Could you check a few things on this model? Use its own coordinates, in mm. Give positions to 0.01 mm unless a question says otherwise; leave off trailing zeros. Loops run counter-clockwise (first coordinate to the right, second up) from the corner with the lowest first, then second, coordinate; pieces in that order, holes last. Notation, with made-up numbers: (26, -37) - (35, -37) arc R21 ccw to (35, -9) - close; hole circle Ø4 at (-18, 71). An arc over 180 degrees is marked (long way). Write each question's results on one line, items separated by ' | '. Start each with the question number.
(1) Suppose I cut it at A-A (y = 0). Count the separate pieces of the cut face and the enclosed holes in it, and give its area (3 significant figures).
(2) Suppose I cut it at B-B (x = 25.4). Please give me the cut outline in (y, z), and give its area (3 significant figures).
(3) For pin 1 (1.2 mm diameter, centred on x = 20, z = -0.5, fed in from +Y); pin 2 (1.2 mm diameter, centred on y = 25, z = -0.5, fed in from +X); pin 3 (1.2 mm diameter, centred on y = 27.5, z = 0.5, fed in from -X), each with a flat end and sliding along its axis, tell me the tip position at first contact or that it passes through.
(4) I need wall thicknesses on line 1 (Y direction, x = 0, z = 0); line 2 (Y direction, x = 1.5, z = -0.5); line 3 (Y direction, x = 21, z = 0.95). Which ranges of each line are inside material? Lowest first, please.
from build123d import *

# Parameters (mm, degrees)
SKETCH1_R           = 2.5
BOSS_EXTRUDE1_DEPTH = 2.5


with BuildPart() as part:
    # Sketch1 → Boss-Extrude1 (new body)
    with BuildSketch(Plane(origin=(0, 0, -1.25), x_dir=(-1, 0, 0), z_dir=(0, 0, -1))):
        Polygon((12.7, 12.7), (12.7, 50.546), (6.35, 56.896), (-6.35, 56.896), (-12.7, 50.546), (-12.7, 12.7), (-37.846, 12.7), (-44.196, 6.35), (-44.196, -6.35), (-37.846, -12.7), (37.846, -12.7), (44.196, -6.35), (44.196, 6.35), (37.846, 12.7), align=None)
        with Locations((0, 50.8)):
            Circle(SKETCH1_R, mode=Mode.SUBTRACT)
        with Locations((0, 38.1)):
            Circle(SKETCH1_R, mode=Mode.SUBTRACT)
        with Locations((-38.1, 0)):
            Circle(SKETCH1_R, mode=Mode.SUBTRACT)
        with Locations((-25.4, 0)):
            Circle(SKETCH1_R, mode=Mode.SUBTRACT)
        with Locations((-12.7, 0)):
            Circle(SKETCH1_R, mode=Mode.SUBTRACT)
        Circle(SKETCH1_R, mode=Mode.SUBTRACT)
        with Locations((12.7, 0)):
            Circle(SKETCH1_R, mode=Mode.SUBTRACT)
        with Locations((38.1, 0)):
            Circle(SKETCH1_R, mode=Mode.SUBTRACT)
        with Locations((25.4, 0)):
            Circle(SKETCH1_R, mode=Mode.SUBTRACT)
        with Locations((0, 12.7)):
            Circle(SKETCH1_R, mode=Mode.SUBTRACT)
        with Locations((0, 25.4)):
            Circle(SKETCH1_R, mode=Mode.SUBTRACT)
    extrude(amount=-BOSS_EXTRUDE1_DEPTH)


solid = part.part
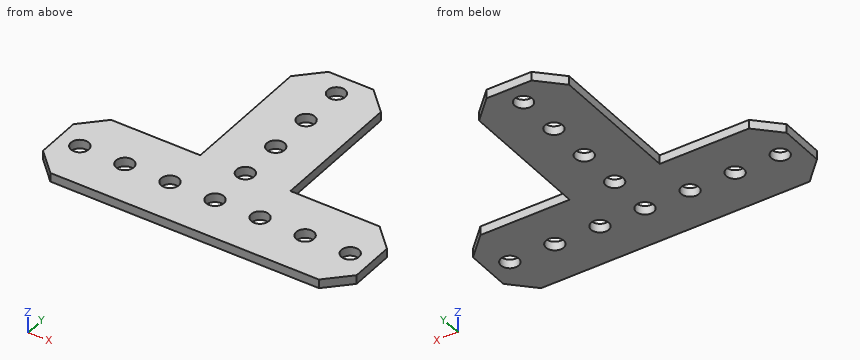
Output values:
1) separate pieces: 8 | enclosed holes: 0 | area: 133 mm2
2) outline: (-12.7, -1.25) - (-2.5, -1.25) - (-2.5, 1.25) - (-12.7, 1.25) - close; (2.5, -1.25) - (12.7, -1.25) - (12.7, 1.25) - (2.5, 1.25) - close | area: 51.0 mm2
3) pin 1: y = 12.7 | pin 2: x = 12.7 | pin 3: x = -12.7
4) line 1: -12.7 to -2.5, 2.5 to 10.2, 15.2 to 22.9, 27.9 to 35.6, 40.6 to 48.3, 53.3 to 56.9 | line 2: -12.7 to -2, 2 to 10.7, 14.7 to 23.4, 27.4 to 36.1, 40.1 to 48.8, 52.8 to 56.9 | line 3: -12.7 to 12.7
